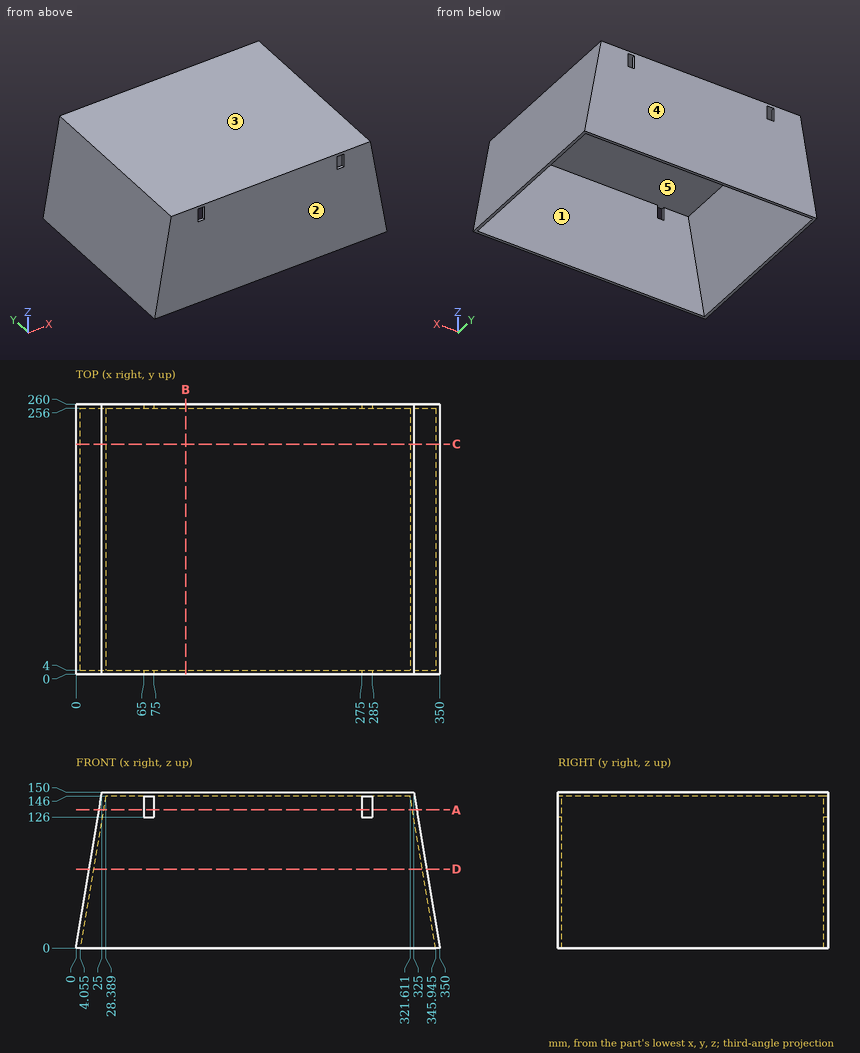
Study the drawing (mm; zero at the part's minimum x, y, z) and answer. A direction names the side the tool comes from. Round coordinates to 2 decimals unless told otherwise and drop trailing zeros. Write each loop counter-clockwise with the first axis right and the second up, starting at its lowest first coordinate (ties: lowest second). Pieces come first, ordered by that corner, then holes.
1) Straight lines are drawn through the part: line 1 (Y direction, x = 186.5, z = 105); line 2 (Z direction, x = 298, y = 66); line 3 (X direction, y = 61, z = 27) (1 decimal). For each, find the intervals that lie inside material, in ascending order.
2) Given pin 1 Ø10 at (x, z) = (206, 33) entering from -Y; pin 2 Ø2 at (y, z) = (1, 132) entering from +X; pin 3 Ø3 at (y, z) = (3, 133.5) entering from -X; pin 4 Ø1.5 at (y, z) = (111.5, 72.5) entering from +X, each flat-ended and moving along its own axis, determine where each tip first touches the part or whether it passes through.
3) A tool of negligible diameter and unlimited length cuts with its end or side. For the marked faces 1 and 2, from which of +Z, -Z, +X, -X, +Y, -Y can it reach the whole face along a straight path? Write none if from no direction.
4) A cutting plane is placed at A-A (z = 133). Give the vertices of the cut face in (x, y), plus the area to 3 significant figures.
5) A cutting plane is placed at B-B (x = 105.5). Give the vertices of the cut face in (y, z).
6) The mould has two halves that part along Y. Classify the marked faces 3, 4 and 5: pulls with the +Y half, pulls with the -Y half, needs draft (parallel to the pull), parting line crosses it, or undercut.
7) A cutting plane is placed at D-D (z = 76). Give the vertices of the cut face in (x, y), plus the area to 3 significant figures.
8) A cutting plane is placed at C-C (y = 221.5). Give the vertices of the cut face in (x, z) (1 decimal).
Completed:
1. line 1: y = 0 to 4, 256 to 260
1. line 2: z = 146 to 150
1. line 3: x = 4.5 to 8.6, 341.4 to 345.5
2. pin 1: stops at y = 0
2. pin 2: stops at x = 328.17
2. pin 3: stops at x = 22
2. pin 4: stops at x = 338.04
3. face 1: -Z
3. face 2: +Z, -Z, +X, -X, -Y
4. outline: (22.17, 0) - (65, 0) - (65, 4) - (26.22, 4) - (26.22, 256) - (65, 256) - (65, 260) - (22.17, 260) - close; (75, 0) - (275, 0) - (275, 4) - (75, 4) - close; (75, 256) - (275, 256) - (275, 260) - (75, 260) - close; (285, 0) - (327.83, 0) - (327.83, 260) - (285, 260) - (285, 256) - (323.78, 256) - (323.78, 4) - (285, 4) - close
4. area: 4,330 mm2
5. outline: (0, 0) - (4, 0) - (4, 146) - (256, 146) - (256, 0) - (260, 0) - (260, 150) - (0, 150) - close
6. face 3: needs draft
6. face 4: pulls with the +Y half
6. face 5: undercut
7. outline: (12.67, 0) - (337.33, 0) - (337.33, 260) - (12.67, 260) - close; hole (16.72, 4) - (333.28, 4) - (333.28, 256) - (16.72, 256) - close
7. area: 4,640 mm2
8. outline: (0, 0) - (4.1, 0) - (28.4, 146) - (321.6, 146) - (345.9, 0) - (350, 0) - (325, 150) - (25, 150) - close
